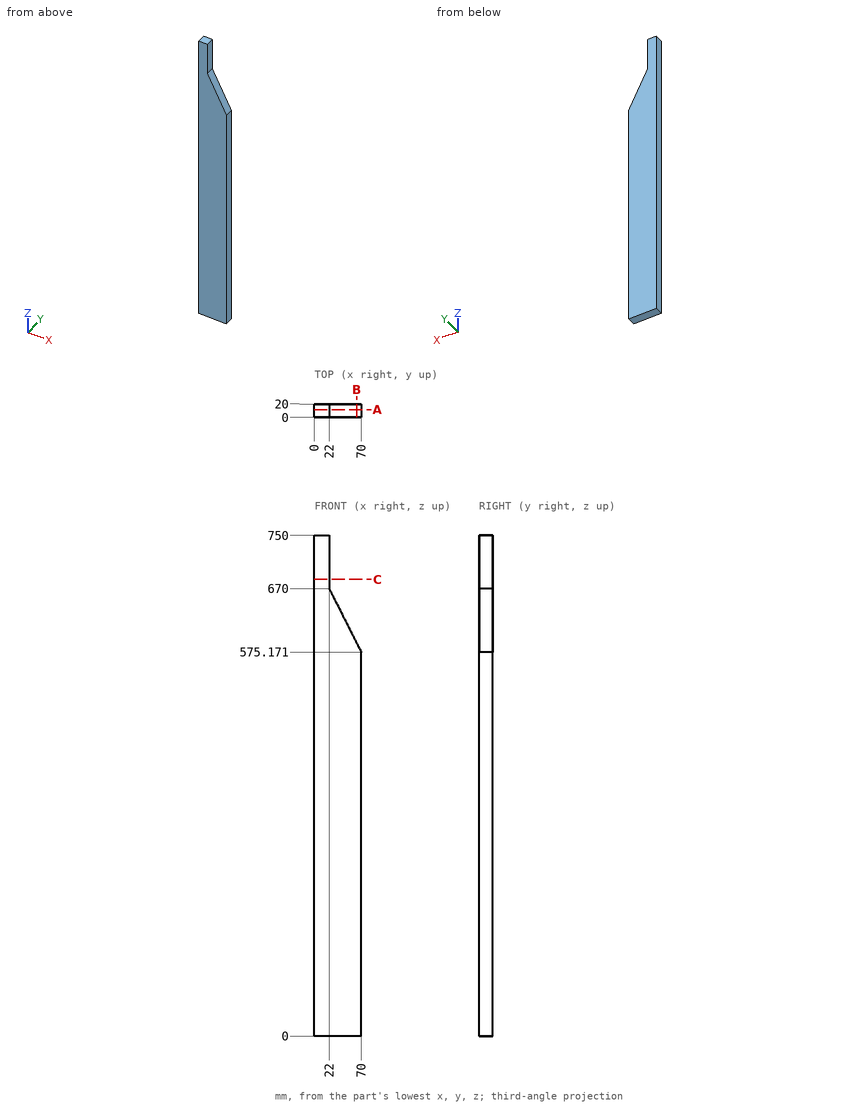
Verification items for this drawing (mm, ordinates from the low corner). Round coordinates to 2 decimals unless told otherwise and drop trailing zeros. Order: outer loops, then holes, each group sorted by start corner. A loop starts at its lowest first (then second) coordinate and runs counter-clockwise, first axis right, second up. Notation, with made-up numbers: (76.25, 51.5) - (113.25, 51.5) arc R13 ccw to (113.25, 57.5) - close; hole circle Ø4 at (-18.5, 74). An arc over 180 degrees is marked (long way). Use CSV: the item, a comma, the result in double quotes. Start each with the question number.
1) Section check B-B, the plane x = 63. Record the cut outline in (y, z).
2) Section check C-C, the plane z = 684. Record the cut outline in (x, y), plus the area to 3 significant figures.
3) Section check A-A, the plane y = 11.75. Record the cut outline in (x, z), plus the area to 3 significant figures.
4) Go/stop test with flat-tipped pins: P1, Ø6, axis at x = 60, y = 9.5, coming from the +Z side (1 decimal); P2, Ø6, axis at y = 12.5, z = 596, coming from the +X side (1 decimal); P3, Ø12, axis at y = 7.5, z = 660, coming from the +X side. Record where each tip stops, or that it passes through.
5) Thickness scan on L1, parallel to Z at x = 55, y = 2 (1 decimal); L2, parallel to Z at x = 59.5, y = 17 (1 decimal); L3, parallel to X at y = 11.5, z = 577 (1 decimal). Record the ranges inside material, lowest first.
Answers:
1,outline,"(0, 0) - (20, 0) - (20, 589) - (0, 589) - close"
2,outline,"(0, 0) - (22, 0) - (22, 20) - (0, 20) - close"
2,area,"440 mm²"
3,outline,"(0, 0) - (70, 0) - (70, 575.17) - (22, 670) - (22, 750) - (0, 750) - close"
3,area,"46,400 mm²"
4,P1,"stops at z = 600.9"
4,P2,"stops at x = 61"
4,P3,"stops at x = 30.1"
5,L1,"z = 0 to 604.8"
5,L2,"z = 0 to 595.9"
5,L3,"x = 0 to 69.1"
